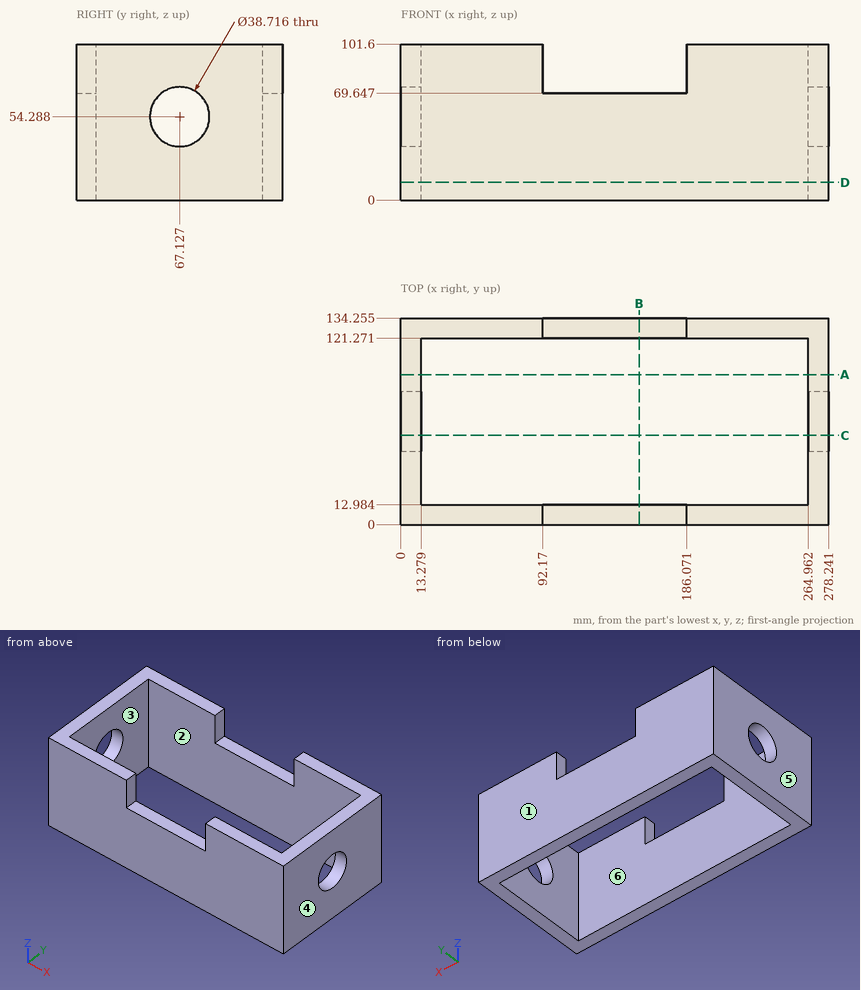
Input: dimensioned drawing with shaded views. Units: mm. Origin: part minimum x, y, z. A direction names the side the tool comes from. Give positions to 0.01 mm unless a question says otherwise; leave off trailing zeros. Loops run counter-clockwise (first coordinate to the right, second up) from the corner with the lowest first, then second, coordinate; pieces in that order, holes last. Notation, with made-up numbers: (83.25, -8) -> (111.25, -8) arc R14 cw to (111.25, 13) -> close; hole circle Ø9 at (78.25, 40.5). An arc over 180 degrees is marked (long way). Use a Markdown table: item, result. Add a question column.
1) Pull-direction query (X, two-part tool) for the marked faces 1, 2, 3 and 4; classes: +X half, -X half, draft (parallel to the pull), parting line (faces both ways), or undercut.
2) Section query C-C, the plane y = 58. Return the cut outline in (x, z), then the cut area to 3 significant figures.
3) Line query: line 1 along Y through (x, z) = (50.5, 49) (1 decimal); line 2 along X through (y, z) = (87.5, 44). Output: solid intervals per line, ascending. Write a range as [from, to].
4) Reachability of the marked faces 5 and 6 from +Z, -Z, +X, -X, +Y, -Y: full face, straight path, thin tool, end or side. Return the list, or none.
5) Section query B-B, the plane x = 155. Return the cut outline in (y, z) (1 decimal), then the cut area to 3 significant figures.
6) First-contact query: pin 1 (4 mm diameter, centred on x = 145, y = 4.5, fed in from +Z). Flat tip, straight axial feed; report the tip coordinate or a pass-through.
7) Section query A-A, the plane y = 97.5. Return the cut outline in (x, z), then the cut area to 3 significant figures.
8) Section query D-D, the plane z = 11.5. Return the cut outline in (x, y) (1 decimal).
Numbers:
| question | item | result |
|---|---|---|
| 1 | face 1 | draft |
| 1 | face 2 | undercut |
| 1 | face 3 | undercut |
| 1 | face 4 | +X half |
| 2 | outline | (0, 0) -> (13.28, 0) -> (13.28, 37.22) -> (0, 37.22) -> close; (0, 71.36) -> (13.28, 71.36) -> (13.28, 101.6) -> (0, 101.6) -> close; (264.96, 0) -> (278.24, 0) -> (278.24, 37.22) -> (264.96, 37.22) -> close; (264.96, 71.36) -> (278.24, 71.36) -> (278.24, 101.6) -> (264.96, 101.6) -> close |
| 2 | area | 1,790 mm2 |
| 3 | line 1 | y = [0, 13], [121.3, 134.3] |
| 3 | line 2 | x = [0, 13.28], [264.96, 278.24] |
| 4 | face 5 | +Z, -Z, -X, +Y, -Y |
| 4 | face 6 | +Z, -Z |
| 5 | outline | (0, 0) -> (13, 0) -> (13, 69.6) -> (0, 69.6) -> close; (121.3, 0) -> (134.3, 0) -> (134.3, 69.6) -> (121.3, 69.6) -> close |
| 5 | area | 1,810 mm2 |
| 6 | pin 1 | stops at z = 69.65 |
| 7 | outline | (0, 0) -> (13.28, 0) -> (13.28, 101.6) -> (0, 101.6) -> close; (264.96, 0) -> (278.24, 0) -> (278.24, 101.6) -> (264.96, 101.6) -> close |
| 7 | area | 2,700 mm2 |
| 8 | outline | (0, 0) -> (278.2, 0) -> (278.2, 134.3) -> (0, 134.3) -> close; hole (13.3, 13) -> (265, 13) -> (265, 121.3) -> (13.3, 121.3) -> close |
